```python
from build123d import *

# Parameters (mm, degrees)
F0_W     = 430
F0_H     = 630
F1_DEPTH = 9
F2_W     = 330
F2_H     = 140
F2_W_2   = 100
F2_H_2   = 100
F2_W_3   = 80
F3_DEPTH = 25


with BuildPart() as f1:
    # F0 (on Front) → F1 (new body)
    with BuildSketch(Plane.XZ):
        with Locations((-215, 315)):
            Rectangle(F0_W, F0_H)
    extrude(amount=F1_DEPTH)

    # F2 (on face) → F3 (cut)
    with BuildSketch(Plane(origin=(0, 0, 0), x_dir=(-1, 0, 0), z_dir=(0, 1, 0))):
        with Locations((215, 120)):
            Rectangle(F2_W, F2_H)
        with Locations((270, 370)):
            Rectangle(F2_W_2, F2_H_2)
        with Locations((80, 460)):
            Rectangle(F2_W_3, F2_H)
    extrude(amount=-F3_DEPTH, mode=Mode.SUBTRACT)


solid = f1.part
```
Geometry check sheet. Reference: the model listing, model coordinates, mm. Give positions to 0.01 mm unless a question says otherwise; leave off trailing zeros. Loops run counter-clockwise (first coordinate to the right, second up) from the corner with the lowest first, then second, coordinate; pieces in that order, holes last. Notation, with made-up numbers: M 87.5,63 L 144.5,63 A10 ccw 144.5,69 Z; hole C -13.5,33.25 d4. An arc over 180 degrees is marked long. Write item = value, one per line.
(1) Sectioned sample at A-A, the plane z = 350. Record the cut outline in (x, y), plus the area to 3 significant figures.
Answer below:
outline = M -430,-9 L -320,-9 L -320,0 L -430,0 Z; M -220,-9 L 0,-9 L 0,0 L -220,0 Z
area = 2,970 mm2
(2) Sectioned sample at B-B, the plane x = -82.5. Record the cut outline in (y, z).
Answer below:
outline = M -9,0 L 0,0 L 0,50 L -9,50 Z; M -9,190 L 0,190 L 0,390 L -9,390 Z; M -9,530 L 0,530 L 0,630 L -9,630 Z
(3) Sectioned sample at C-C, the plane y = -4.75. Record the cut outline in (x, z).
Answer below:
outline = M -430,0 L 0,0 L 0,630 L -430,630 Z; hole M -380,50 L -50,50 L -50,190 L -380,190 Z; hole M -320,320 L -220,320 L -220,420 L -320,420 Z; hole M -120,390 L -40,390 L -40,530 L -120,530 Z
(4) Material ranges on line 1 (Z direction, x = -270.5, y = -8.25); line 2 (Z direction, x = -116.5, y = -4); line 3 (X direction, y = -5.75, z = 402.5), recorded low to high. Write a range as [from, to].
Answer below:
line_1 = [0, 50], [190, 320], [420, 630]
line_2 = [0, 50], [190, 390], [530, 630]
line_3 = [-430, -320], [-220, -120], [-40, 0]
(5) Sectioned sample at D-D, the plane z = 121. Record the cut outline in (x, y).
Answer below:
outline = M -430,-9 L -380,-9 L -380,0 L -430,0 Z; M -50,-9 L 0,-9 L 0,0 L -50,0 Z
